Can you work these out from the drawing? Everything is in mm from the part's minimum corner. A direction names the side the tool comes from. Round coordinates to 2 decimals unless told otherwise and drop trailing zeros. Loops run counter-clockwise (first coordinate to the right, second up) from the corner with the lowest first, then second, coordinate; pieces in that order, holes last. Notation, with made-up numbers: (75.25, 4) -> (81.25, 4) arc R18 cw to (81.25, 26) -> close; hole circle Ø2 at (46.5, 62.5). An arc over 180 degrees is marked (long way). One line per item, written item: value.
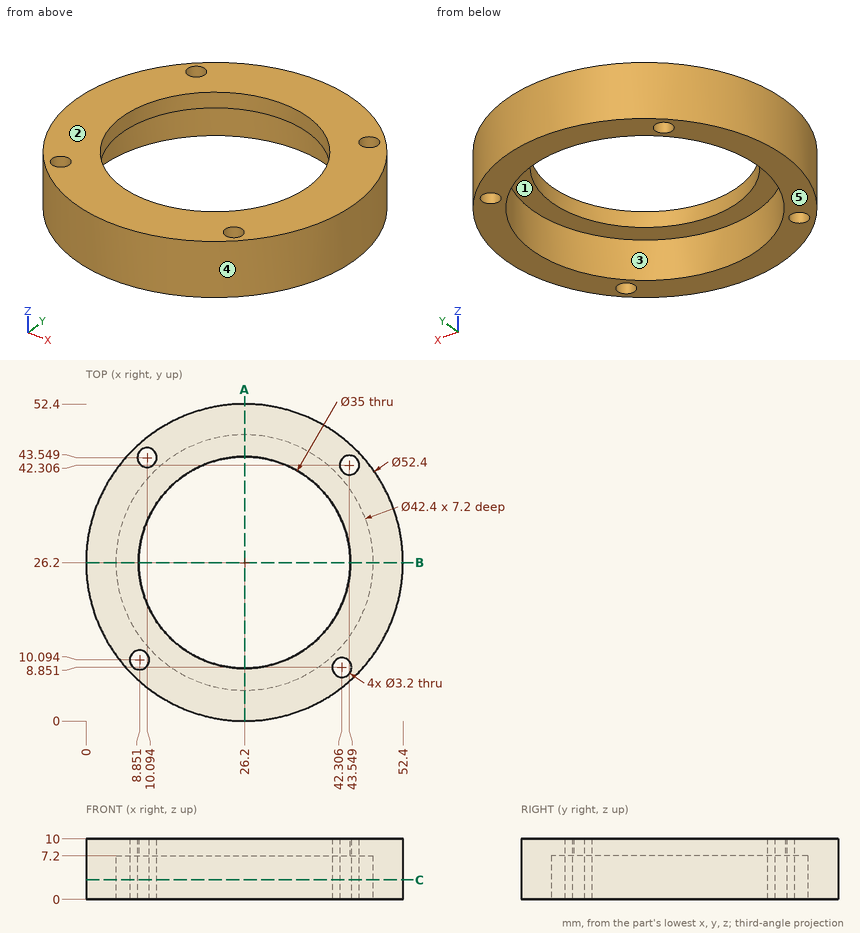
(1) If we section it at A-A, the plane x = 26.2: Please give me the cut outline in (y, z).
Recorded:
outline: (0, 0) -> (5, 0) -> (5, 7.2) -> (8.7, 7.2) -> (8.7, 10) -> (0, 10) -> close; (43.7, 7.2) -> (47.4, 7.2) -> (47.4, 0) -> (52.4, 0) -> (52.4, 10) -> (43.7, 10) -> close
(2) For the marked faces 1 and 2, which set-ups out of +Z, -Z, +X, -X, +Y, -Y let a thin tool reach every point of the face, with its end or its side?
Recorded:
face 1: -Z
face 2: +Z, +X, -X, +Y, -Y
(3) I'm going to push flat-ended pins straight in: pin 1 Ø10 at (x, y) = (19, 36) entering from -Z; pin 2 Ø6 at (x, z) = (37, 5) entering from +Y; pin 3 Ø1 at (x, z) = (27.5, 8) entering from -Y; pin 4 Ø2 at (y, z) = (32.5, 7) entering from -X. Where does each tip first touch, or does it pass through?
Recorded:
pin 1: through
pin 2: y = 51.21
pin 3: y = 0.01
pin 4: x = 0.54
(4) If we section it at C-C, the plane z = 3.25: Please give me the cut outline in (x, y).
Recorded:
outline: circle Ø52.4 at (26.2, 26.2); hole circle Ø42.4 at (26.2, 26.2); hole circle Ø3.2 at (8.85, 10.09); hole circle Ø3.2 at (10.09, 43.55); hole circle Ø3.2 at (42.31, 8.85); hole circle Ø3.2 at (43.55, 42.31)
(5) If I drill on L1, parallel to Y at x = 26.2, z = 9.35; L2, parallel to Y at x = 41.5, z = 4.25 (1 decimal); L3, parallel to Y at x = 10.5, z = 1.75 (1 decimal), over which ranges is the centre line in solid material (lowest first)?
Recorded:
L1: 0 to 8.7, 43.7 to 52.4
L2: 4.9 to 7.5, 10.2 to 11.5, 40.9 to 47.5
L3: 5.2 to 12, 40.4 to 42, 45.1 to 47.2
(6) Thinking about a two-plate mould opening in X: for the marked faces 3, 4 and 5, which applies, released by +X, released by -X, zero draft, split by the parting line, or undercut?
Recorded:
face 3: undercut
face 4: split by the parting line
face 5: zero draft
